Design review of the part built by this model. Coordinates are the model's own, in mm. A direction names the side the tool comes from. Round coordinates to 2 decimals unless told otherwise and drop trailing zeros. Order: outer loops, then holes, each group sorted by start corner. A loop starts at its lowest first (then second) coordinate and runs counter-clockwise, first axis right, second up. Notation, with made-up numbers: (55.5, 29) - (86.5, 29) arc R28 cw to (86.5, 59) - close; hole circle Ø11 at (-5, 87). An arc over 180 degrees is marked (long way). Use CSV: the item, a comma, the result in double quotes.
Autodesk Inventor part; units mm, degrees
ref_plane "YZ Plane" through (0, 0, 0) normal (1, 0, 0) x (0, 1, 0)
ref_plane "XZ Plane" through (0, 0, 0) normal (0, 1, 0) x (-1, 0, 0)
ref_plane "XY Plane" through (0, 0, 0) normal (0, 0, 1) x (1, 0, 0)
sketch "スケッチ6" plane through (0, 0, 0) normal (0, 0, 1) x (1, 0, 0)
  line L0 (0, 0) -> (25, 0)
  line L1 (25, 0) -> (25, 30)
  line L2 (25, 30) -> (0, 30)
  line L3 (0, 30) -> (0, 0)
  circle A0 centre (5, 5) radius 2.5
  circle A1 centre (20, 5) radius 2.5
  dimension "d39" = 5
  dimension "d40" = 5
  dimension "d41" = 5
  dimension "d42" = 5
  dimension "d43" = 15
  dimension "d44" = 5
  dimension "d45" = 5
  dimension "d46" = 30
extrude "押し出し4" add sketch "スケッチ6" along normal blind 5
sketch "スケッチ7" plane through (0, 0, 5) normal (0, 0, 1) x (1, 0, 0)
  line L0 (25, 30) -> (0, 30)
  line L1 (10, 30) -> (15, 30)
  line L2 (15, 30) -> (15, 10)
  line L3 (15, 10) -> (10, 10)
  line L4 (10, 10) -> (10, 30)
  line L5 (25, 0) -> (25, 30)
  line L6 (0, 30) -> (0, 0)
  line L7 (0, 0) -> (25, 0)
  line L8 (10, 30) -> (15, 30)
  line L9 (15, 30) -> (15, 60)
  line L10 (15, 60) -> (10, 60)
  line L11 (10, 60) -> (10, 30)
  dimension "d49" = 5
  dimension "d50" = 10
  dimension "d51" = 10
  dimension "d52" = 10
  dimension "d55" = 30
  dimension "d56" = 5
extrude "押し出し5" add sketch "スケッチ7" along normal blind 10 contours L2 L3 L4 L0 | L0 L11 L10 L9
sketch "スケッチ8" plane through (10, 30, 5) normal (-1, 0, 0) x (0, 0, 1)
  line L0 (10, 30) -> (10, -20)
  line L1 (0, 30) -> (10, 30)
  line L2 (0, -20) -> (10, -20)
  point P0 (-5, -30)
  point P1 (3.1, 11.5)
  point P2 (3.1, 23.5)
  dimension "d57" = 6.9
  dimension "d58" = 6.9
  dimension "d59" = 12
  dimension "d60" = 6.5
  dimension "d61" = 31.5
hole "穴3" at (10, 41.5, 8.1) at (10, 53.5, 8.1) direction (1, 0, 0) diameter 5 depth 8
sketch "スケッチ9" plane through (0, 0, 5) normal (0, 0, 1) x (1, 0, 0)
  line L0 (10, 30) -> (0, 30)
  line L1 (0, 30) -> (7, 30)
  line L2 (7, 30) -> (7, 10)
  line L3 (7, 10) -> (0, 10)
  line L4 (0, 10) -> (0, 30)
  line L5 (25, 0) -> (25, 30)
  line L6 (25, 30) -> (18, 30)
  line L7 (18, 30) -> (18, 10)
  line L8 (18, 10) -> (25, 10)
  line L9 (25, 10) -> (25, 30)
  point P0 (0, 0)
  point P1 (5, 30)
  point P2 (18, 20)
  point P3 (7, 20)
  dimension "d70" = 20
  dimension "d72" = 7
  dimension "d73" = 7
extrude "押し出し6" cut sketch "スケッチ9" against normal blind 10
fillet "フィレット4" radius 1 15 edges at (7, 30, 2.5) (12.5, 60, 5) (12.5, 60, 15) (12.5, 10, 15) (7, 10, 2.5) (0, 10, 2.5) (0, 0, 2.5) (18, 30, 2.5) (18, 10, 2.5) (25, 10, 2.5) (25, 0, 2.5) (10, 20, 5) (12.5, 30, 5) (15, 20, 5) (12.5, 10, 5)
sketch "スケッチ10" plane through (0, 0, 5) normal (0, 0, 1) x (1, 0, 0)
  line L0 (9, 30) -> (9, 9)
  line L1 (9, 30) -> (8, 30)
  arc A0 (8, 30) -> (7, 29) centre (8, 29) ccw
  line L2 (7, 29) -> (7, 11)
  arc A1 (6, 10) -> (7, 11) centre (6, 11) ccw
  line L3 (6, 10) -> (1, 10)
  arc A2 (1, 10) -> (0, 9) centre (1, 9) ccw
  line L4 (0, 9) -> (0, 1)
  arc A3 (0, 1) -> (1, 0) centre (1, 1) ccw
  line L5 (1, 0) -> (24, 0)
  arc A4 (24, 0) -> (25, 1) centre (24, 1) ccw
  line L6 (25, 1) -> (25, 9)
  arc A5 (25, 9) -> (24, 10) centre (24, 9) ccw
  line L7 (24, 10) -> (19, 10)
  arc A6 (18, 11) -> (19, 10) centre (19, 11) ccw
  line L8 (18, 11) -> (18, 29)
  arc A7 (18, 29) -> (17, 30) centre (17, 29) ccw
  line L9 (17, 30) -> (16, 30)
  line L10 (16, 9) -> (16, 30)
  line L11 (9, 9) -> (16, 9)
  circle A8 centre (5, 5) radius 2.5
  circle A9 centre (20, 5) radius 2.5
  line L12 (2, 8) -> (23, 8)
  line L13 (23, 8) -> (23, 2)
  line L14 (23, 2) -> (2, 2)
  line L15 (2, 2) -> (2, 8)
  line L16 (2, 10) -> (2, 0)
  line L17 (24, 10) -> (19, 10)
  line L18 (23, 10) -> (23, 0)
  point P0 (0, 0)
  point P1 (2, 2)
  point P2 (23, 2)
  dimension "d77" = 2
  dimension "d78" = 2
  dimension "d79" = 2
  dimension "d80" = 2
extrude "押し出し7" cut sketch "スケッチ10" against normal blind 4 contours L16 L15 L5 A3 L4 A2 L3 | L18 L7 A5 L6 A4 L5 L13
fillet "フィレット5" radius 1 4 edges at (23, 10, 3) (23, 0, 3) (2, 10, 3) (2, 0, 3)
sketch "スケッチ11" plane through (15, 31, 5) normal (1, 0, 0) x (0, 0, -1)
  line L0 (-7.1, 27) -> (2, 27)
  line L1 (2, 5.5) -> (-7.1, 5.5)
  line L2 (-7.1, 5.5) -> (-7.1, 27)
  line L3 (0, 0) -> (0, 28)
  circle A0 centre (-3.1, 22.5) radius 2.5
  line L4 (-7.1, 27) -> (0.9, 27)
  line L5 (0.9, 27) -> (0.9, 5.5)
  line L6 (0.9, 5.5) -> (-7.1, 5.5)
  line L7 (-7.1, 5.5) -> (-7.1, 27)
  line L8 (-1, 29) -> (-9, 29)
  circle A1 centre (-3.1, 10.5) radius 2.5
  point P0 (5, -31)
  point P1 (0.9, 27)
  point P2 (0, 27)
  point P3 (0, 5.5)
  dimension "d85" = 4
  dimension "d86" = 4
  dimension "d87" = 2
  dimension "d88" = 5
extrude "押し出し8" add sketch "スケッチ11" against normal blind 5 contours L0 L5 L1 L3
fillet "フィレット6" radius 0.5 4 edges at (12.5, 36.5, 5) (12.5, 36.5, 4.1) (12.5, 58, 4.1) (12.5, 58, 5)
equation "\"d42\" = d41"
equation "\"d45\" = d44"
equation "\"d73\" = d72"
equation "\"d86\" = d85"
properties part number "BP_BOX-Support-Bar-Connect1-40" material "ABS プラスチック"
1) Insertion check: pin 1 Ø4 at (x, z) = (18.5, 7.5) entering from -Y; pin 2 Ø2.5 at (x, y) = (13.5, 33.5) entering from -Z; pin 3 Ø1.5 at (x, y) = (11.5, 49) entering from -Z; pin 4 Ø4 at (y, z) = (19.5, 3.5) entering from -X. Each pin has a flat end and moves straight along its axis. Give the tip position at first contact, or say it passes through.
Data:
pin 1,"passes through"
pin 2,"stops at z = 5"
pin 3,"stops at z = 4.1"
pin 4,"stops at x = 7"
2) We need section D-D (y = 53.5). Give the boundary of the cut face in (x, z), then the cut area to 3 significant figures.
Data:
outline,"(10, 4.1) - (15, 4.1) - (15, 5.6) - (10, 5.6) - close; (10, 10.6) - (15, 10.6) - (15, 15) - (10, 15) - close"
area,"29.5 mm2"
3) For faces 1 (the face through (18, 20, 3)), 2 (the face through (15, 35, 11)), 3 (the face through (10, 35, 11)), 4 (the face through (13, 10, 10)), 5 (the face through (23, 5, 3)), list the 3-axis set-ups (+Z, -Z, +X, -X, +Y, -Y) from which the entire face can be reached by the end or side of a thin tool; tool diameter is ignored.
Data:
face 1,"+Z, -Z, +X, +Y"
face 2,"+Z, +X, +Y"
face 3,"+Z, -X, +Y"
face 4,"+Z, +X, -X, -Y"
face 5,"+Z, +X, +Y, -Y"
4) We need section C-C (y = 5). Give the boundary of the cut face in (x, z).
Data:
outline,"(0, 0) - (2.5, 0) - (2.5, 5) - (2, 5) - (2, 1) - (0, 1) - close; (7.5, 0) - (17.5, 0) - (17.5, 5) - (7.5, 5) - close; (22.5, 0) - (25, 0) - (25, 1) - (23, 1) - (23, 5) - (22.5, 5) - close"
5) We need section A-A (z = 8.1). Give the boundary of the cut face in (x, y).
Data:
outline,"(10, 10) - (15, 10) - (15, 39) - (10, 39) - close; (10, 44) - (15, 44) - (15, 51) - (10, 51) - close; (10, 56) - (15, 56) - (15, 60) - (10, 60) - close"
6) The part is to be moulded in two halves that separate along Z. For faces 6 (the face through (12.4, 8.5, 5)), 7 (the face through (2, 5, 3)), 8 (the face through (13, 44, 8)), 9 (the face through (12.5, 53.4, 5.6)), say which applies: +Z half, -Z half, draft (parallel to the pull), parting line (faces both ways), or undercut.
Data:
face 6,"+Z half"
face 7,"draft"
face 8,"undercut"
face 9,"undercut"
7) We need section B-B (x = 5). Give the boundary of the cut face in (y, z), then the cut area to 3 significant figures.
Data:
outline,"(0, 0) - (2.5, 0) - (2.5, 5) - (0, 5) - close; (7.5, 0) - (10, 0) - (10, 5) - (7.5, 5) - close"
area,"25.0 mm2"
8) To check wall thickness, follow L1, parallel to Z at x = 13.45, y = 41.5; L2, parallel to Y at x = 20, z = 2.8; L3, parallel to X at y = 6.5, z = 2. State the ranges of each line that lie inside material, in increasing order. Write a range as from..to.
Data:
L1,"z = 4.1..5.6, 10.6..15"
L2,"y = 0..2.5, 7.5..10"
L3,"x = 2..3, 7..18, 22..23"
